Source: three-view drawing plus pictorial views. Frame: mm from the lowest corner of the part. Round coordinates to 2 decimals unless told otherwise and drop trailing zeros. Write each loop counter-clockwise with the first axis right and the second up, starting at its lowest first coordinate (ties: lowest second). Pieces come first, ordered by that corner, then holes. Notation, with made-up numbers: M 57.25,70 L 75.25,70 A17 ccw 75.25,92 Z; hole C 16.25,8.5 d4. An arc over 180 degrees is marked long. Answer in a Markdown table with one row per item.
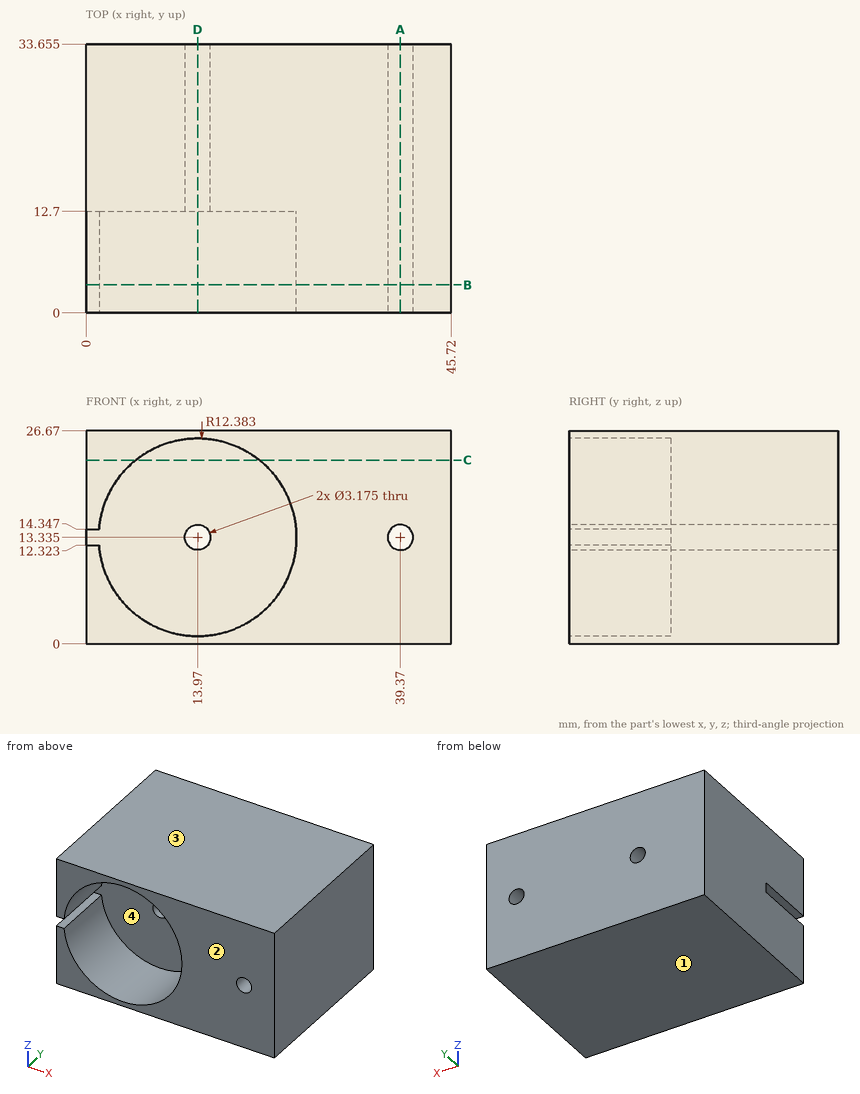
Q1. Pull-direction query (Z, two-part tool) for the marked faces 1, 2, 3 and 4; classes: pulls with the +Z half, pulls with the -Z half, needs draft (parallel to the pull), parting line crosses it, or undercut.
Solutions:
| item | result |
|---|---|
| face 1 | pulls with the -Z half |
| face 2 | needs draft |
| face 3 | pulls with the +Z half |
| face 4 | undercut |
Q2. Section C-C (z = 23). Return loops of the section in (x, y) (1 decimal), and give its area (3 significant figures).
Solutions:
| item | result |
|---|---|
| outline | M 0,0 L 6.2,0 L 6.2,12.7 L 21.7,12.7 L 21.7,0 L 45.7,0 L 45.7,33.7 L 0,33.7 Z |
| area | 1,340 mm2 |
Q3. Section D-D (x = 13.97). Return loops of the section in (y, z) (1 decimal).
Solutions:
| item | result |
|---|---|
| outline | M 0,0 L 33.7,0 L 33.7,11.7 L 12.7,11.7 L 12.7,1 L 0,1 Z; M 0,25.7 L 12.7,25.7 L 12.7,14.9 L 33.7,14.9 L 33.7,26.7 L 0,26.7 Z |
Q4. Section B-B (y = 3.5). Return loops of the section in (x, z) (1 decimal).
Solutions:
| item | result |
|---|---|
| outline | M 0,0 L 45.7,0 L 45.7,26.7 L 0,26.7 L 0,14.3 L 1.6,14.3 A12.4 cw long 1.6,12.3 L 0,12.3 Z; hole C 39.4,13.3 d3.2 |
Q5. Contact query for a flat-ended pin moving along its axis: pin 1 Ø8 at (x, z) = (17.5, 14) entering from -Y. Output: stop coordinate, or through.
Solutions:
| item | result |
|---|---|
| pin 1 | stops at y = 12.7 |
Q6. Section A-A (x = 39.37). Return loops of the section in (y, z) (1 decimal), and give its area (3 significant figures).
Solutions:
| item | result |
|---|---|
| outline | M 0,0 L 33.7,0 L 33.7,11.7 L 0,11.7 Z; M 0,14.9 L 33.7,14.9 L 33.7,26.7 L 0,26.7 Z |
| area | 791 mm2 |
Q7. Material intervals for probe 1 along Y at (x, z) = (19, 10.5) (1 decimal); probe 2 along X at (y, z) = (12.5, 13); probe 3 along Z at (x, y) = (15, 17.5) (1 decimal), sorted ascending.
Solutions:
| item | result |
|---|---|
| probe 1 | y = 12.7 to 33.7 |
| probe 2 | x = 26.35 to 37.82, 40.92 to 45.72 |
| probe 3 | z = 0 to 12.1, 14.5 to 26.7 |
